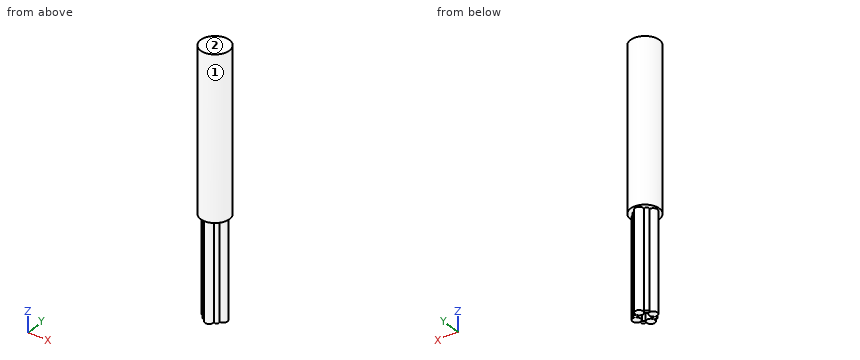
from build123d import *

# Parameters (mm, degrees)
F0_R     = 44.45
F1_DEPTH = 497.84
F2_R     = 12.7
F2_R_2   = 6.35
F3_DEPTH = 304.8


with BuildPart() as f1:
    # F0 (on Top) → F1 (new body)
    with BuildSketch(Plane.XY):
        Circle(F0_R)
    extrude(amount=-F1_DEPTH)

    # F2 (on face) → F3 (join)
    with BuildSketch(Plane(origin=(0, 0, -497.84), x_dir=(1, 0, 0), z_dir=(0, 0, -1))):
        with Locations((0, 25.4)):
            Circle(F2_R)
        with Locations((0, -25.4)):
            Circle(F2_R)
        with Locations((-25.4, 0)):
            Circle(F2_R)
        with Locations((25.4, 0)):
            Circle(F2_R)
        with Locations((-17.960512, 17.960512)):
            Circle(F2_R_2)
        with Locations((17.960512, 17.960512)):
            Circle(F2_R_2)
        with Locations((17.960512, -17.960512)):
            Circle(F2_R_2)
        with Locations((-17.960512, -17.960512)):
            Circle(F2_R_2)
    extrude(amount=F3_DEPTH)


solid = f1.part
Check sheet for the modelled part. Datum: model origin and axes. Units: mm. Face numbers are marked on the shaded views. Round coordinates to 2 decimals unless told otherwise and drop trailing zeros. Order: outer loops, then holes, each group sorted by start corner. A loop starts at its lowest first (then second) coordinate and runs counter-clockwise, first axis right, second up. Notation, with made-up numbers: M 4,35.25 L 15,35.25 A14 ccw 15,52.25 Z; hole C -28,71.5 d9. An arc over 180 degrees is marked long. One line per item, written item: value. Start each with the question number.
1. Scan lines: line 1 along Y through (x, z) = (22.5, -598); line 2 along Y through (x, z) = (-15, -576); line 3 along X through (y, z) = (-1, -695). Record each from-to range of solid material in increasing order.
2. Section check A-A on x = 0. Enter the section's corners in (y, z), and give its area (3 significant figures).
3. Gauge pin test, flat ends, axial feed: P1, Ø4, axis at y = -24, z = -657.5, coming from the +X side; P2, Ø2, axis at x = -0.5, z = -383.5, coming from the +Y side; P3, Ø1, axis at y = -8.5, z = -429, coming from the -X side. Record the tip position at first contact, or that the pin passes through.
4. Release check for a two-part mould opening along Z. For the marked faces 1 and 2 record: released by +Z, released by -Z, zero draft, split by the parting line, or undercut.
5. Section check C-C on z = -179.5. Enter the section's corners in (x, y), and give its area (3 significant figures).
Results found:
1. line 1: -22.4 to -13.52, -12.36 to 12.36, 13.52 to 22.4
1. line 2: -23.58 to -12.34, -7.29 to 7.29, 12.34 to 23.58
1. line 3: -38.06 to -12.74, 12.74 to 38.06
2. outline: M -44.45,-497.84 L -38.1,-497.84 L -38.1,-802.64 L -12.7,-802.64 L -12.7,-497.84 L 12.7,-497.84 L 12.7,-802.64 L 38.1,-802.64 L 38.1,-497.84 L 44.45,-497.84 L 44.45,0 L -44.45,0 Z
2. area: 59,700 mm^2
3. P1: x = 22.86
3. P2: y = 44.45
3. P3: x = -43.72
4. face 1: zero draft
4. face 2: released by +Z
5. outline: C 0,0 d88.9
5. area: 6,210 mm^2
